Work out the finished part from the listing and answer in its coordinate system (mm). Give positions to 0.01 mm unless a question says otherwise; leave off trailing zeros. Order: outer loops, then holes, each group sorted by start corner. A loop starts at its lowest first (then second) coordinate and runs counter-clockwise, first axis right, second up. Notation, with made-up numbers: (-25, 58.25) -> (-8, 58.25) arc R8 cw to (-8, 70.25) -> close; hole circle Ø4 at (58, 70.25). An arc over 180 degrees is marked (long way). Answer as CSV lines item,"result". Start each with the question number.
1. A cutting plane is placed at C-C (y = 61). Give the vertices of the cut face in (x, z), then the cut area to 3 significant figures.
2. Find the intervals of material crossed by L1, parallel to Y at x = 63, z = 0.8; L2, parallel to Y at x = 0, z = 1.6; L3, parallel to X at y = -59.5, z = 2.15, in increasing order.
3. A cutting plane is placed at A-A (x = 0). Give the vertices of the cut face in (y, z).
4. Flat-ended cylindrical pins translate along their axes: pin 1 (1.5 mm diameter, centred on x = 20.5, z = 1.5, fed in from +Y); pin 2 (3.5 mm diameter, centred on x = 63, y = 60.5, fed in from +Z). Find the tip coordinate at first contact, or state that the pin passes through.
5. A cutting plane is placed at B-B (z = 0.6). Give the vertices of the cut face in (x, y).
6. A cutting plane is placed at D-D (y = -5.5). Give the vertices of the cut face in (x, z).
from build123d import *

# Parameters (mm, degrees)
SKETCH_1_R          = 1.6
EXTRUDE_1_DEPTH     = 2.5
SKETCH_2_R          = 20
CUT_EXTRUDE_1_DEPTH = 23
SKETCH_3_R          = 3.5
CUT_EXTRUDE_2_DEPTH = 1.2


with BuildPart() as part:
    # 草图1 → 凸台-拉伸1 (new body)
    with BuildSketch(Plane.XY):
        with BuildLine():
            Line((68.5, 66), (33, 66))
            ThreePointArc((33, 66), (0, 33), (-33, 66))
            Line((-33, 66), (-68.5, 66))
            Line((-68.5, 66), (-68.5, 30.44898712))
            ThreePointArc((-68.5, 30.44898712), (-43.537948759, 21.765123634), (-32.954411074, -2.452684221))
            ThreePointArc((-32.954411074, -2.452684221), (-43.537948759, -26.670492075), (-68.5, -35.354355562))
            Line((-68.5, -35.354355562), (-68.5, -66))
            Line((-68.5, -66), (-33, -66))
            ThreePointArc((-33, -66), (0, -33), (33, -66))
            Line((33, -66), (68.5, -66))
            Line((68.5, -66), (68.5, -30.44898712))
            ThreePointArc((68.5, -30.44898712), (32.954411074, 2.452684221), (68.5, 35.354355562))
            Line((68.5, 35.354355562), (68.5, 66))
        make_face()
        with Locations((-63.310606061, -61)):
            Circle(SKETCH_1_R, mode=Mode.SUBTRACT)
        with Locations((63.310606061, -61)):
            Circle(SKETCH_1_R, mode=Mode.SUBTRACT)
        with Locations((-63.310606061, 61)):
            Circle(SKETCH_1_R, mode=Mode.SUBTRACT)
        with Locations((63.310606061, 61)):
            Circle(SKETCH_1_R, mode=Mode.SUBTRACT)
    extrude(amount=EXTRUDE_1_DEPTH)

    # 草图2 → 切除-拉伸1 (cut)
    with BuildSketch(Plane.XY.offset(2.5)):
        Circle(SKETCH_2_R)
    extrude(amount=-CUT_EXTRUDE_1_DEPTH, mode=Mode.SUBTRACT)

    # 草图3 → 切除-拉伸2 (cut)
    with BuildSketch(Plane.XY.offset(2.5)):
        with Locations((63.310606061, -61)):
            Circle(SKETCH_3_R)
        with Locations((63.310606061, 61)):
            Circle(SKETCH_3_R)
        with Locations((-63.310606061, 61)):
            Circle(SKETCH_3_R)
        with Locations((-63.310606061, -61)):
            Circle(SKETCH_3_R)
    extrude(amount=-CUT_EXTRUDE_2_DEPTH, mode=Mode.SUBTRACT)


solid = part.part
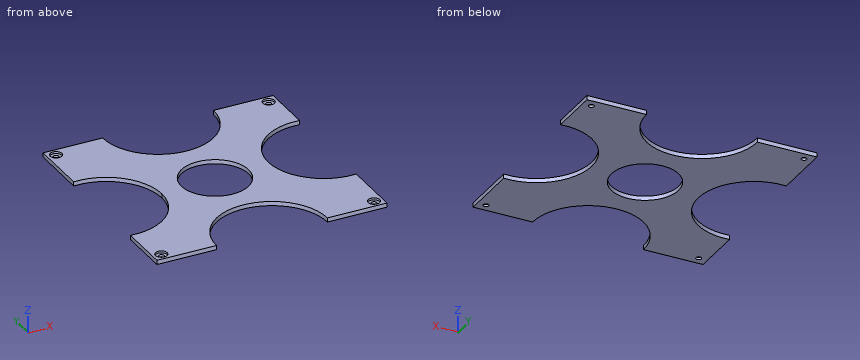
Answer sheet:
1,outline,"(-68.5, 0) -> (-64.91, 0) -> (-64.91, 1.3) -> (-66.81, 1.3) -> (-66.81, 2.5) -> (-68.5, 2.5) -> close; (-61.71, 0) -> (-32.62, 0) -> (-32.62, 2.5) -> (-59.81, 2.5) -> (-59.81, 1.3) -> (-61.71, 1.3) -> close; (32.62, 0) -> (61.71, 0) -> (61.71, 1.3) -> (59.81, 1.3) -> (59.81, 2.5) -> (32.62, 2.5) -> close; (64.91, 0) -> (68.5, 0) -> (68.5, 2.5) -> (66.81, 2.5) -> (66.81, 1.3) -> (64.91, 1.3) -> close"
1,area,"154 mm^2"
2,L1,"y = -66 to -62.57, -59.43 to -30.41, 35.32 to 59.43, 62.57 to 66"
2,L2,"y = -33 to -20, 20 to 33"
2,L3,"x = -68.5 to -66.47, -60.15 to -32.35, 32.35 to 60.15, 66.47 to 68.5"
3,outline,"(-33, 0) -> (-20, 0) -> (-20, 2.5) -> (-33, 2.5) -> close; (20, 0) -> (33, 0) -> (33, 2.5) -> (20, 2.5) -> close"
4,pin 1,"stops at y = 40.75"
4,pin 2,"stops at z = 1.3"
5,outline,"(-68.5, -66) -> (-33, -66) arc R33 cw to (33, -66) -> (68.5, -66) -> (68.5, -30.45) arc R33 cw (long way) to (68.5, 35.35) -> (68.5, 66) -> (33, 66) arc R33 cw to (-33, 66) -> (-68.5, 66) -> (-68.5, 30.45) arc R33 cw (long way) to (-68.5, -35.35) -> close; hole circle Ø3.2 at (-63.31, -61); hole circle Ø3.2 at (-63.31, 61); hole circle Ø40 at (0, 0); hole circle Ø3.2 at (63.31, -61); hole circle Ø3.2 at (63.31, 61)"
6,outline,"(-33.1, 0) -> (-19.23, 0) -> (-19.23, 2.5) -> (-33.1, 2.5) -> close; (19.23, 0) -> (33.93, 0) -> (33.93, 2.5) -> (19.23, 2.5) -> close"
